The listing builds one solid part. Answer for the finished solid, in the listing's coordinates (mm). Give positions to 0.01 mm unless a question says otherwise; leave off trailing zeros. Write each loop counter-clockwise with the first axis right and the second up, starting at its lowest first coordinate (ties: lowest second). Pieces come first, ordered by that corner, then holes. Notation, with made-up numbers: (39, -10) - (49, -10) arc R22 cw to (49, 25) - close; hole circle Ø8 at (-33.75, 73). An arc over 180 degrees is marked (long way). Write each question's results on one line, items separated by ' | '. Start each with the question number.
Q1. Section B-B (y = 205) is taken. Determine the outline of the cut face in (x, z), plus the area to 3 significant figures.
Q2. Find the intervals of material crossed by probe 1 along X at (y, z) = (-32, 798); probe 2 along X at (y, z) = (-165.5, 649); probe 3 along Y at (x, z) = (-353, 687.5), in increasing order.
Q3. Flat-ended cylindrical pins translate along their axes: pin 1 Ø12 at (x, y) = (234.5, 33.5) entering from +Z; pin 2 Ø10 at (x, y) = (-39, -356) entering from +Z. Find the tip coordinate at first contact, or state that the pin passes through.
Q4. Section D-D (x = -370.5) is taken. Determine the outline of the cut face in (y, z).
Q5. Section A-A (x = 140) is taken. Determine the outline of the cut face in (y, z), plus the area to 3 significant figures.
Q6. Section C-C (z = 874.5) is taken. Determine the outline of the cut face in (x, y).
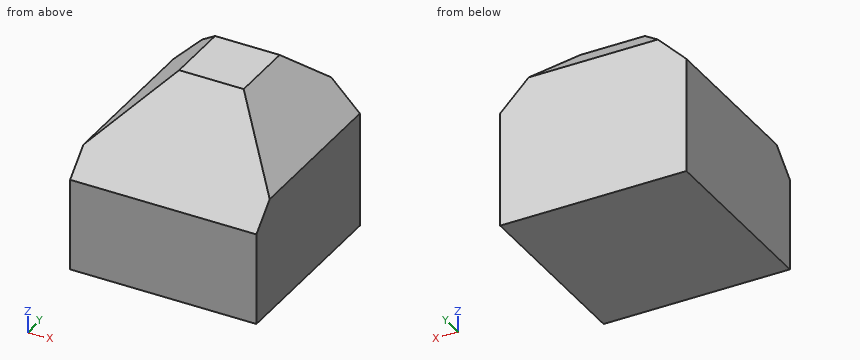
```python
from build123d import *

# Parameters (mm, degrees)
F0_W     = 1010
F0_H     = 1010
F1_DEPTH = 956
F3_DEPTH = 1010
F4_DEPTH = 1010
F6_DEPTH = 1010


with BuildPart() as f1:
    # F0 (on Top) → F1 (new body)
    with BuildSketch(Plane.XY):
        Rectangle(F0_W, F0_H)
    extrude(amount=F1_DEPTH)

    # F2 (on face) → F3 (cut)
    with BuildSketch(Plane(origin=(-505, 0, 0), x_dir=(0, -1, 0), z_dir=(-1, 0, 0))):
        Polygon((-505, 956), (-505, 781), (-316, 956), align=None)
    extrude(amount=-F3_DEPTH, mode=Mode.SUBTRACT)

    # F2 (on face) → F4 (cut)
    with BuildSketch(Plane(origin=(-505, 0, 0), x_dir=(0, -1, 0), z_dir=(-1, 0, 0))):
        Polygon((505, 956), (35, 956), (505, 500), align=None)
    extrude(amount=-F4_DEPTH, mode=Mode.SUBTRACT)

    # F5 (on face) → F6 (cut)
    with BuildSketch(Plane.XZ.offset(505)):
        Polygon((-505, 626), (-175, 956), (-505, 956), align=None)
        Polygon((505, 626), (505, 956), (175, 956), align=None)
    extrude(amount=-F6_DEPTH, mode=Mode.SUBTRACT)


solid = f1.part
```
Answers below:
1) outline: (-505, 0) - (505, 0) - (505, 626) - (175, 956) - (-175, 956) - (-505, 626) - close | area: 857,000 mm2
2) probe 1: x = -333 to 333 | probe 2: x = -482 to 482 | probe 3: y = -311.74 to 505
3) pin 1: stops at z = 902.5 | pin 2: stops at z = 649.41
4) outline: (-505, 0) - (505, 0) - (505, 760.5) - (-236.5, 760.5) - (-505, 500) - close
5) outline: (-505, 0) - (505, 0) - (505, 781) - (316, 956) - (-35, 956) - (-505, 500) - close | area: 842,000 mm2
6) outline: (-256.5, -119) - (256.5, -119) - (256.5, 404.02) - (-256.5, 404.02) - close
